```python
from build123d import *

# Parameters (mm, degrees)
F0_W      = 44.1452
F0_H      = 9.2456
F1_DEPTH  = 59.055
F2_W      = 44.1452
F2_H      = 9.7089702415
F3_DEPTH  = 6.096
F5_DEPTH  = 81.026
F6_DEPTH  = 82.296
F8_DEPTH  = 67.564
F9_W      = 40.8686
F9_H      = 7.366
F10_DEPTH = 15.748
F11_W     = 6.735065354
F11_H     = 7.366
F12_DEPTH = 12.7


with BuildPart() as f1:
    # F0 (on Front) → F1 (new body)
    with BuildSketch(Plane.XZ):
        Rectangle(F0_W, F0_H)
    extrude(amount=-F1_DEPTH)

    # F2 (on face) → F3 (join)
    with BuildSketch(Plane.XY.offset(4.6228)):
        with Locations((0, 54.2005148792)):
            Rectangle(F2_W, F2_H)
    extrude(amount=F3_DEPTH)

    # F4 (on face) → F5 (cut)
    with BuildSketch(Plane.XZ):
        Polygon((-9.4742, -2.3368), (-11.6586, -4.6228), (18.796, -4.6228), (16.9926, -2.0828), (18.796, -2.0828), (18.796, 2.7432), (-11.6586, 2.7432), (-11.6586, -2.3368), align=None)
    extrude(amount=-F5_DEPTH, mode=Mode.SUBTRACT)

    # F4 (on face) → F6 (cut)
    with BuildSketch(Plane.XZ):
        Polygon((-18.796, -4.6228), (-13.716, -4.6228), (-13.716, 2.7432), (-18.796, 2.7432), (-18.796, -2.0828), (-16.9926, -2.0828), align=None)
        Polygon((-9.4742, -2.3368), (-11.6586, -4.6228), (18.796, -4.6228), (16.9926, -2.0828), (18.796, -2.0828), (18.796, 2.7432), (-11.6586, 2.7432), (-11.6586, -2.3368), align=None)
    extrude(amount=-F6_DEPTH, mode=Mode.SUBTRACT)

    # F7 (on face) → F8 (cut)
    with BuildSketch(Plane(origin=(-22.0726, 0, 0), x_dir=(0, -1, 0), z_dir=(-1, 0, 0))):
        Polygon((-52.1785840392, 10.7188), (-49.3460297585, 4.6228), (-49.3460297585, 10.7188), align=None)
    extrude(amount=-F8_DEPTH, mode=Mode.SUBTRACT)

    # F9 (on face) → F10 (cut)
    with BuildSketch(Plane(origin=(0, 59.055, 0), x_dir=(-1, 0, 0), z_dir=(0, 1, 0))):
        with Locations((1.6383, -0.9398)):
            Rectangle(F9_W, F9_H)
    extrude(amount=-F10_DEPTH, mode=Mode.SUBTRACT)

    # F11 (on face) → F12 (cut)
    with BuildSketch(Plane.XZ):
        with Locations((-10.348467323, -0.9398)):
            Rectangle(F11_W, F11_H)
    extrude(amount=-F12_DEPTH, mode=Mode.SUBTRACT)


with BuildPart() as f13_1:
    # F13: instance of F1
    add(f1.part.mirror(Plane.YZ))


with BuildPart() as f15_1:
    # F15: instance of F13_1
    add(f13_1.part.mirror(Plane.YZ))


solid = f15_1.part
```
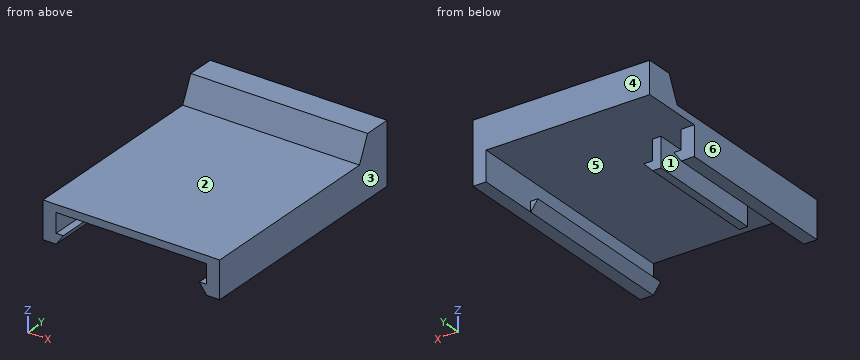
CAD build for the part. Positions are in the model's coordinates, mm. Face numbers are marked on the shaded views. A direction names the side the tool comes from. Coordinates: 2 decimals unless noted, no trailing zeros. Order: outer loops, then holes, each group sorted by start corner. A loop starts at its lowest first (then second) coordinate and runs counter-clockwise, first axis right, second up.
(1) Pin check, flat tips, straight feed: pin 1 Ø4.5 at (x, z) = (-12.5, -2) entering from +Y; pin 2 Ø0.5 at (x, z) = (17.5, -3.5) entering from +Y; pin 3 Ø3.5 at (x, z) = (-12, -1) entering from -Y; pin 4 Ø0.9 at (x, y) = (18, 23) entering from +Z. Stop position of each tip, or through.
Solution:
pin 1: stops at y = 43.31
pin 2: passes through
pin 3: stops at y = 12.7
pin 4: stops at z = 4.62
(2) Mould opens along X. For the marked faces 4, 5 and 6 say: released by +X, released by -X, zero draft, split by the parting line, or undercut.
Solution:
face 4: zero draft
face 5: undercut
face 6: released by -X
(3) Saw through at A-A, the plane z = -0.75. Write the cut outline in (x, y) (3 decimals), and give its area (3 significant figures).
Solution:
outline: (-22.073, 0) - (-18.796, 0) - (-18.796, 43.307) - (-22.073, 43.307) - close; (-13.716, 12.7) - (-11.659, 12.7) - (-11.659, 43.307) - (-13.716, 43.307) - close; (18.796, 0) - (22.073, 0) - (22.073, 59.055) - (18.796, 59.055) - close
area: 398 mm2
(4) Drill centre lines: L1, parallel to X at y = 15, z = -0.5; L2, parallel to X at y = 23, z = -3; L3, parallel to Z at x = -2.5, y = 7.5. Where is each one in solid material? Low to high.
Solution:
L1: x = -22.07 to -18.8, -13.72 to -11.66, 18.8 to 22.07
L2: x = -22.07 to -17.64, -13.72 to -10.11, 17.64 to 22.07
L3: z = 2.74 to 4.62
(5) Saw through at B-B, the plane y = 8. Write the cut outline in (x, z).
Solution:
outline: (-22.07, -4.62) - (-18.8, -4.62) - (-16.99, -2.08) - (-18.8, -2.08) - (-18.8, 2.74) - (18.8, 2.74) - (18.8, -2.08) - (16.99, -2.08) - (18.8, -4.62) - (22.07, -4.62) - (22.07, 4.62) - (-22.07, 4.62) - close
(6) Saw through at C-C, the plane x = 4. Write the cut outline in (y, z) (3 decimals).
Solution:
outline: (0, 2.743) - (59.055, 2.743) - (59.055, 10.719) - (52.179, 10.719) - (49.346, 4.623) - (0, 4.623) - close
(7) Saw through at D-D, the plane y = 45. Write the cut outline in (x, z), and give its area (3 significant figures).
Solution:
outline: (-22.07, 2.74) - (18.8, 2.74) - (18.8, -4.62) - (22.07, -4.62) - (22.07, 4.62) - (-22.07, 4.62) - close
area: 107 mm2
(8) Which spindle directions (+Z, -Z, +X, -X, +Y, -Y) get a long thin tool onto all of the face, cutting with end or side? Do the marked faces 1, 2 and 3. Say none if no direction does.
Solution:
face 1: -Z, +Y, -Y
face 2: +Z, +X, -X, -Y
face 3: +Z, -Z, +X, +Y, -Y
